Autodesk Inventor part; units mm, degrees
ref_plane "YZ Plane" through (0, 0, 0) normal (1, 0, 0) x (0, 1, 0)
ref_plane "XZ Plane" through (0, 0, 0) normal (0, 1, 0) x (-1, 0, 0)
ref_plane "XY Plane" through (0, 0, 0) normal (0, 0, 1) x (1, 0, 0)
sketch "Esquisse1" plane through (0, 0, 0) normal (1, 0, 0) x (0, 1, 0)
  line L0 (0, 0) -> (155, 0)
  line L1 (155, 0) -> (155, -155)
  line L2 (155, -155) -> (0, -155)
  line L3 (0, -155) -> (0, 0)
  line L4 (5, -5) -> (150, -5)
  line L5 (150, -5) -> (150, -150)
  line L6 (150, -150) -> (5, -150)
  line L7 (5, -150) -> (5, -5)
  dimension "d0" = 155
  dimension "d1" = 155
  dimension "d2" = 145
  dimension "d3" = 145
extrude "Extrusion1" add sketch "Esquisse1" along normal blind 13
sketch "Esquisse2" plane through (13, 0, 0) normal (1, 0, 0) x (0, 0, -1)
  line L0 (2.5, 2.5) -> (152.5, 2.5)
  line L1 (152.5, 2.5) -> (152.5, 152.5)
  line L2 (152.5, 152.5) -> (2.5, 152.5)
  line L3 (2.5, 152.5) -> (2.5, 2.5)
  line L4 (150, 5) -> (5, 5)
  line L5 (5, 5) -> (150, 5)
  line L6 (150, 5) -> (150, 150)
  line L7 (150, 150) -> (5, 150)
  line L8 (5, 150) -> (5, 5)
  point P0 (0, 0)
  point P1 (155, 155)
  dimension "d7" = 150
  dimension "d8" = 150
extrude "Extrusion2" cut sketch "Esquisse2" against normal blind 3
properties part number "rebord1515"
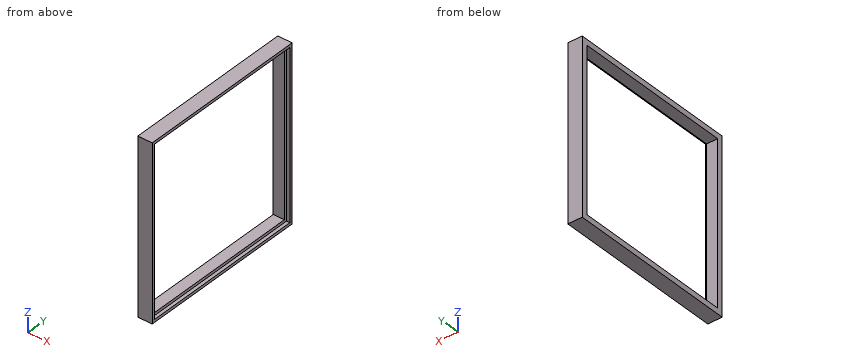
Could you check a few things on this model? Use its own coordinates, in mm. Give positions to 0.01 mm unless a question says otherwise; leave off trailing zeros. Write each loop counter-clockwise with the first axis right and the second up, starting at its lowest first coordinate (ties: lowest second). Pieces come first, ordered by that corner, then holes. Notation, with made-up numbers: (41.25, 36.5) - (49.25, 36.5) arc R13 cw to (49.25, 53.5) - close; hole circle Ø7 at (-29.75, 73). An arc over 180 degrees is marked (long way). One line per item, written item: value. Start each with the question number.
Item 1: Imagine slicing it at C-C, the plane x = 5.25. List the corners of the cut face in (y, z) for me.
Item 2: Please list where these lines run through material, in increasing order: line 1 (Y direction, x = 2.75, z = -71); line 2 (Y direction, x = 11.5, z = -137.5); line 3 (Z direction, x = 5.25, y = 78.5). Write a range as from..to.
Item 3: Imagine slicing it at A-A, the plane z = -118.5. List the corners of the cut face in (x, y) for me.
Item 4: Imagine slicing it at B-B, the plane y = 34. List the corners of the cut face in (x, z) for me.
Geometry says:
1. outline: (0, -155) - (155, -155) - (155, 0) - (0, 0) - close; hole (5, -150) - (150, -150) - (150, -5) - (5, -5) - close
2. line 1: 0..5, 150..155
2. line 2: 0..2.5, 152.5..155
2. line 3: -155..-150, -5..0
3. outline: (0, 0) - (13, 0) - (13, 2.5) - (10, 2.5) - (10, 5) - (0, 5) - close; (0, 150) - (10, 150) - (10, 152.5) - (13, 152.5) - (13, 155) - (0, 155) - close
4. outline: (0, -155) - (13, -155) - (13, -152.5) - (10, -152.5) - (10, -150) - (0, -150) - close; (0, -5) - (10, -5) - (10, -2.5) - (13, -2.5) - (13, 0) - (0, 0) - close
